Input: part model. Units: mm. Frame: model coordinates. A direction names the side the tool comes from. Coordinates: 2 decimals unless noted, no trailing zeros. Write each loop counter-clockwise with the first axis right and the second up, starting at its lowest first coordinate (ties: lowest second). Pieces come first, ordered by that corner, then holes. Notation, with made-up numbers: M 36.5,6.25 L 86.5,6.25 A34 ccw 86.5,39.25 Z; hole C 36.5,80.25 d3. An arc over 180 degrees is marked long. Answer as a JSON object with one key per item and string values. Group by question number.
from build123d import *

# Parameters (mm, degrees)
F1_DEPTH = 6
F2_R     = 1


with BuildPart() as f1:
    # F0 (on Top) → F1 (new body)
    with BuildSketch(Plane.XY):
        with BuildLine():
            Line((-4.25, 0), (-9.994602, 4.594337))
            ThreePointArc((-9.994602, 4.594337), (5.443818, -9.558496), (1.147387, 10.939996))
            Line((1.147387, 10.939996), (1.622562, 3.928078))
            ThreePointArc((1.622562, 3.928078), (2.362902, -3.53259), (-4.25, 0))
        make_face()
    extrude(amount=F1_DEPTH)

    # F2
    f2_edges = [f1.edges().sort_by_distance(p)[0] for p in [
        (5.443818, -9.558496, 6),
        (2.362902, -3.53259, 6),
        (2.362902, -3.53259, 0),
        (5.443818, -9.558496, 0),
        (-7.122301, 2.297168, 0),
        (-9.994602, 4.594337, 3),
        (-7.122301, 2.297168, 6),
        (1.384974, 7.434037, 0),
        (1.147387, 10.939996, 3),
        (1.384974, 7.434037, 6),
    ]]
    fillet(f2_edges, radius=F2_R)


solid = f1.part
Q1. Pin query (flat end, axial travel): pin 1 Ø1 at (x, z) = (4.5, 3) entering from -Y; pin 2 Ø2 at (x, z) = (2.5, 2.5) entering from -Y; pin 3 Ø7 at (x, y) = (0, 0) entering from +Z; pin 4 Ø1.5 at (x, z) = (5.5, 2) entering from +Y. Return the tip coordinate at first contact, or that it passes through.
Q2. Section A-A, the plane z = 1.5. Return the cut outline in (x, y), and give its area (3 significant figures).
Q3. Line query: line 1 (Y direction, x = 0, z = 3.3); line 2 (Y direction, x = 3.75, z = 3.25); line 3 (Y direction, x = 3, z = 1.25). Output: solid intervals per line, ascending. Write a range as from..to.
Q4. Access query for faces 1 (the cylindrical face through (-6.8, 1.67, 0.3)), 2 (the cylindrical face through (-9.83, 3.92, 3.03)), 3 (the cylindrical face through (-6.8, 1.67, 5.7)). Directions: +Z, -Z, +X, -X, +Y, -Y. A direction counts if a zero-diameter tool reaches every point of the face in a straight line with its end or side. Return the directions, or none.
Q5. Draft query along X for faces 4 (the flat face through (4, -4, 6)), 5 (the flat face through (-6.556, 1.844, 2.972)), 6 (the cylindrical face through (5.17, -9.71, 2.97)). Return one class per face: released by +X, released by -X, zero draft, split by the parting line, or undercut.
Filled in:
{
 "1": {"pin 1": "y = -10.25", "pin 2": "y = -10.9", "pin 3": "through", "pin 4": "y = 9.92"},
 "2": {"outline": "M -10.51,3.26 A11 ccw long 2.45,10.72 A1 ccw 1.23,9.68 L 1.62,3.93 A4.25 cw long -4.25,0 L -8.93,3.74 A1 ccw Z", "area": "249 mm^2"},
 "3": {"line 1": "-11..-4.25", "line 2": "-10.34..-2, 2..10.34", "line 3": "-10.58..-3.01, 3.01..10.58"},
 "4": {"face 1": "-Z, +Y", "face 2": "+Z, -Z, +Y", "face 3": "+Z, +Y"},
 "5": {"face 4": "zero draft", "face 5": "undercut", "face 6": "split by the parting line"}
}
